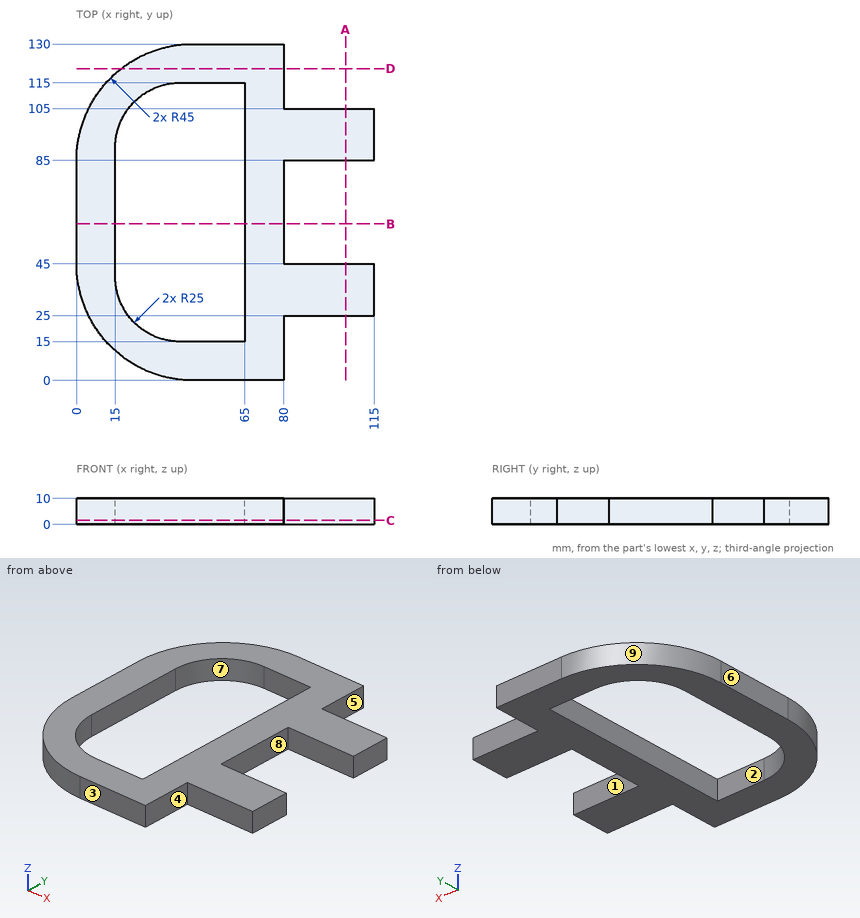
Print and shaded views of the part. All mm, measured from the part's lowest x, y and z. A direction names the side the tool comes from. Coordinates: 2 decimals unless noted, no trailing zeros. Write each loop counter-clockwise with the first axis right and the second up, starting at its lowest first coordinate (ties: lowest second). Pieces come first, ordered by that corner, then holes.
(1) Drill centre lines: probe 1 along Y at (x, z) = (57, 5); probe 2 along X at (y, z) = (80, 0.5); probe 3 along Y at (x, z) = (103, 8.25). Where is each one in solid material? Low to high.
(2) Cut at B-B, the plane y = 60.5. List the corners of the cut face in (x, z).
(3) Cut at A-A, the plane x = 104. List the corners of the cut face in (y, z).
(4) Two-plate mould, pull along Y, no slides. Class the marked faces 6, 7, 8 and 9: +Y half, -Y half, draft (parallel to the pull), parting line (faces both ways), or undercut.
(5) Cut at D-D, the plane y = 120.5. List the corners of the cut face in (x, z), and give its area (3 significant figures).
(6) Flat gauge pins, fed straight in: pin 1 (2 mm diameter, centred on x = 90.5, z = 7.5, fed in from +Y); pin 2 (5 mm diameter, centred on y = 41.5, z = 6, fed in from -X); pin 3 (5 mm diameter, centred on x = 99.5, z = 4, fed in from -Y). Where does each tip first touch, or does it go through?
(7) 3-axis set-ups, long thin cutter, end or side, ignore diameter. For the marked faces 1, 2, 3, 4 and 5: which of +Z, -Z, +X, -X, +Y, -Y reach the whole face in a straight line?
(8) Cut at C-C, the plane z = 1.5. List the corners of the cut face in (x, y), and give its area (3 significant figures).
Geometry says:
1. probe 1: y = 0 to 15, 115 to 130
1. probe 2: x = 0 to 15, 65 to 80
1. probe 3: y = 25 to 45, 85 to 105
2. outline: (0, 0) - (15, 0) - (15, 10) - (0, 10) - close; (65, 0) - (80, 0) - (80, 10) - (65, 10) - close
3. outline: (25, 0) - (45, 0) - (45, 10) - (25, 10) - close; (85, 0) - (105, 0) - (105, 10) - (85, 10) - close
4. face 6: draft
4. face 7: undercut
4. face 8: undercut
4. face 9: +Y half
5. outline: (17.35, 0) - (80, 0) - (80, 10) - (17.35, 10) - close
5. area: 627 mm2
6. pin 1: stops at y = 105
6. pin 2: stops at x = 0.01
6. pin 3: stops at y = 25
7. face 1: +Z, -Z, +X
7. face 2: +Z, -Z
7. face 3: +Z, -Z, +X, -X, -Y
7. face 4: +Z, -Z, +X, -Y
7. face 5: +Z, -Z, +X, +Y
8. outline: (0, 45) arc R45 ccw to (45, 0) - (80, 0) - (80, 25) - (115, 25) - (115, 45) - (80, 45) - (80, 85) - (115, 85) - (115, 105) - (80, 105) - (80, 130) - (45, 130) arc R45 ccw to (0, 85) - close; hole (15, 40) arc R25 ccw to (40, 15) - (65, 15) - (65, 115) - (40, 115) arc R25 ccw to (15, 90) - close
8. area: 6,200 mm2
